Source: three-view drawing plus pictorial views. Frame: mm from the lowest corner of the part. A direction names the side the tool comes from. Round coordinates to 2 decimals unless told otherwise and drop trailing zeros. Write each loop counter-clockwise with the first axis right and the second up, starting at its lowest first coordinate (ties: lowest second). Pieces come first, ordered by that corner, then holes. Notation, with made-up numbers: (-12, 42.5) - (1, 42.5) arc R13 cw to (1, 50.5) - close; hole circle Ø9 at (12.5, 64). An arc over 180 degrees is marked (long way). Write each question's results on one line, items separated by ' | '.
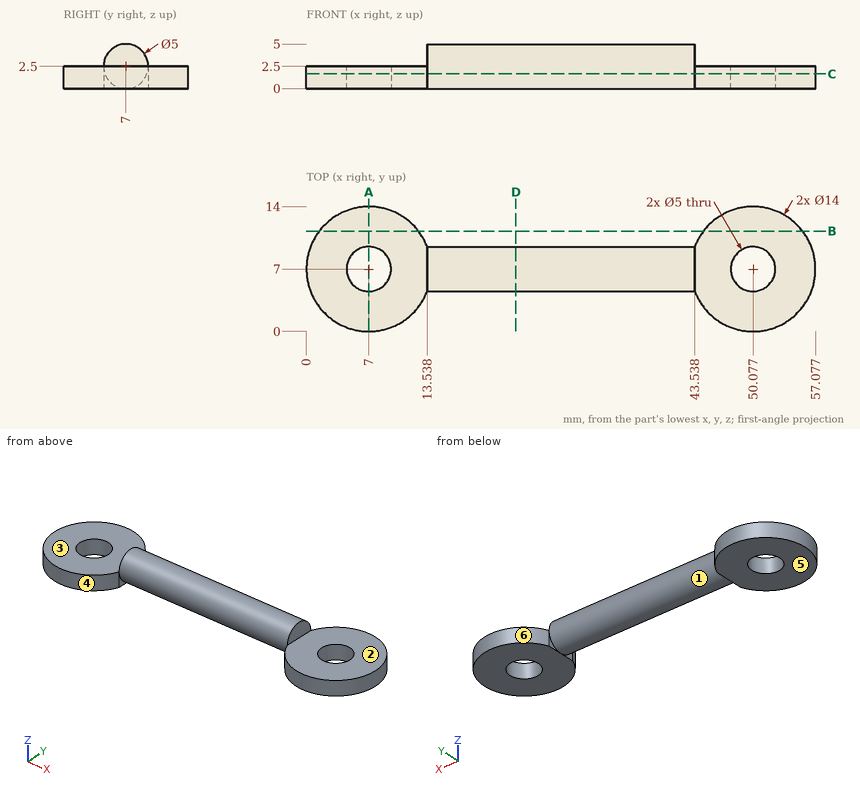
Q1. Section query B-B, the plane y = 11.25. Return loops of the section in (x, z) (1 decimal).
Answer block:
outline: (1.4, 0) - (12.6, 0) - (12.6, 2.5) - (1.4, 2.5) - close; (44.5, 0) - (55.6, 0) - (55.6, 2.5) - (44.5, 2.5) - close
Q2. Section query C-C, the plane z = 1.65. Return loops of the section in (x, y).
Answer block:
outline: (13.54, 4.5) - (13.54, 4.65) - (43.54, 4.65) - (43.54, 4.5) arc R7 ccw (long way) to (43.54, 9.5) - (43.54, 9.35) - (13.54, 9.35) - (13.54, 9.5) arc R7 ccw (long way) to start; hole circle Ø5 at (7, 7); hole circle Ø5 at (50.08, 7)
Q3. Ray query, line 1 along X through (y, z) = (7, 1); line 2 along Y through (x, z) = (7, 1.55); line 3 along X through (y, z) = (7.75, 1.8) (1 decimal). Return the intervals inside material, ascending.
Answer block:
line 1: 0 to 4.5, 9.5 to 47.58, 52.58 to 57.08 | line 2: 0 to 4.5, 9.5 to 14 | line 3: 0 to 4.6, 9.4 to 47.7, 52.5 to 57
Q4. Pin query (flat end, axial travel): pin 1 (4.5 mm diameter, centred on x = 50.08, y = 7, fed in from +Z); pin 2 (7 mm diameter, centred on x = 53, y = 4, fed in from +Z); pin 3 (8 mm diameter, centred on x = 12.5, y = 3, fed in from +Z); pin 4 (0.8 mm diameter, centred on y = 6.5, z = 3.5, fed in from -X). Return the tip coordinate at first contact, or that it passes through.
Answer block:
pin 1: through | pin 2: z = 2.5 | pin 3: z = 5 | pin 4: x = 13.54
Q5. Access query for the marked faces 1, 2 and 3. Directions: +Z, -Z, +X, -X, +Y, -Y. A direction counts if a zero-diameter tool reaches every point of the face in a straight line with its end or side. Return the directions, or none.
Answer block:
face 1: none | face 2: +Z, +X, +Y, -Y | face 3: +Z, -X, +Y, -Y
Q6. Section query D-D, the plane x = 23.5. Return loops of the section in (y, z), plus the area to 3 significant figures.
Answer block:
outline: circle Ø5 at (7, 2.5) | area: 19.6 mm2
Q7. Mould query, pull axis X, two halves, no side actions, for the marked faces 4, 5 and 6. Classes: pulls with the +X half, pulls with the -X half, needs draft (parallel to the pull), parting line crosses it, or undercut.
Answer block:
face 4: undercut | face 5: needs draft | face 6: undercut
Q8. Section query A-A, the plane x = 7. Return loops of the section in (y, z).
Answer block:
outline: (0, 0) - (4.5, 0) - (4.5, 2.5) - (0, 2.5) - close; (9.5, 0) - (14, 0) - (14, 2.5) - (9.5, 2.5) - close
